```python
from build123d import *

# Parameters (mm, degrees)
F0_R     = 1.43764
F0_R_2   = 3.175
F1_DEPTH = 2.286


with BuildPart() as f1:
    # F0 (on Front) → F1 (new body)
    with BuildSketch(Plane.XZ):
        with BuildLine():
            Line((-11.43, 0), (-17.212507, -11.5316))
            ThreePointArc((-17.212507, -11.5316), (-16.638674, -19.900319), (-8.316873, -20.955))
            ThreePointArc((-8.316873, -20.955), (0, -19.152777), (8.316873, -20.955))
            ThreePointArc((8.316873, -20.955), (16.638674, -19.900319), (17.212507, -11.5316))
            Line((17.212507, -11.5316), (12.146577, -1.429014))
            ThreePointArc((12.146577, -1.429014), (12.173853, -0.810849), (12.714209, -0.509375))
            Line((12.714209, -0.509375), (33.02, -0.509375))
            ThreePointArc((33.02, -0.509375), (35.941, 2.411625), (33.02, 5.332625))
            Line((33.02, 5.332625), (8.437909, 5.332625))
            ThreePointArc((8.437909, 5.332625), (6.409691, 5.70754), (4.543451, 6.585822))
            ThreePointArc((4.543451, 6.585822), (2.379373, 7.639017), (0, 8.001))
            ThreePointArc((0, 8.001), (-0.739302, 7.953795), (-1.474639, 7.863933))
            ThreePointArc((-1.474639, 7.863933), (-7.494188, 5.250922), (-11.43, 0))
        make_face()
        with Locations((-11.8364, -15.367)):
            Circle(F0_R, mode=Mode.SUBTRACT)
        with Locations((11.8364, -15.367)):
            Circle(F0_R, mode=Mode.SUBTRACT)
        with Locations((1.27, 3.2512)):
            Circle(F0_R_2, mode=Mode.SUBTRACT)
    extrude(amount=F1_DEPTH)


solid = f1.part
```
Design review of the part built by this model. Coordinates are the model's own, in mm. A direction names the side the tool comes from. Round coordinates to 2 decimals unless told otherwise and drop trailing zeros. Write each loop counter-clockwise with the first axis right and the second up, starting at its lowest first coordinate (ties: lowest second). Pieces come first, ordered by that corner, then holes. Notation, with made-up numbers: (36.5, -32.75) -> (46.5, -32.75) arc R25 cw to (46.5, -15.75) -> close; hole circle Ø8 at (48, 88). An arc over 180 degrees is marked (long way). Answer in a Markdown table with one row per item.
Q1. To check wall thickness, follow L1, parallel to Z at x = 12, y = -0.6; L2, parallel to Z at x = 13, y = -1.5; L3, parallel to X at y = -1.9, z = -15.75. State the ranges of each line that lie inside material, in increasing order. Write a range as [from, to].
The answers:
| item | result |
|---|---|
| L1 | [-21.97, -16.8], [-13.94, 5.33] |
| L2 | [-21.87, -16.21], [-14.52, -3.13], [-0.51, 5.33] |
| L3 | [-18.43, -13.22], [-10.45, 10.45], [13.22, 18.43] |
Q2. Take a section at A-A, the plane x = 14. State the section outline as (y, z) points.
The answers:
| item | result |
|---|---|
| outline | (-2.29, -21.61) -> (0, -21.61) -> (0, -5.13) -> (-2.29, -5.13) -> close; (-2.29, -0.51) -> (0, -0.51) -> (0, 5.33) -> (-2.29, 5.33) -> close |
Q3. Clearance check with flat-ended pins moving along their axes: pin 1 Ø2.5 at (x, z) = (11.84, -15.37) entering from +Y; pin 2 Ø1.1 at (x, y) = (26, -1.5) entering from -Z. State where each tip first meets the part, or that it passes through.
The answers:
| item | result |
|---|---|
| pin 1 | through |
| pin 2 | z = -0.51 |
Q4. Take a section at C-C, the plane z = 1. State the section outline as (x, y) points, then the cut area to 3 significant figures.
The answers:
| item | result |
|---|---|
| outline | (-10.97, -2.29) -> (-0.97, -2.29) -> (-0.97, 0) -> (-10.97, 0) -> close; (3.51, -2.29) -> (35.58, -2.29) -> (35.58, 0) -> (3.51, 0) -> close |
| area | 96.2 mm² |
Q5. For faces 1 (the face through (21, -1, 5.333)), 2 (the face through (23, -1, -0.509)), 3 (the face through (-14.281, -1.127, -5.685)), list the 3-axis set-ups (+Z, -Z, +X, -X, +Y, -Y) from which the entire face can be reached by the end or side of a thin tool; tool diameter is ignored.
The answers:
| item | result |
|---|---|
| face 1 | +Z, +X, +Y, -Y |
| face 2 | +X, +Y, -Y |
| face 3 | +Z, -X, +Y, -Y |
Q6. Take a section at D-D, the plane z = -5.75. State the section outline as (x, y) points.
The answers:
| item | result |
|---|---|
| outline | (-14.31, -2.29) -> (14.31, -2.29) -> (14.31, 0) -> (-14.31, 0) -> close |
Q7. Take a section at B-B, the plane y = -0.8. Count the separate pieces of the cut face and the enclosed holes in it, then the cut area to 3 significant figures.
The answers:
| item | result |
|---|---|
| separate pieces | 1 |
| enclosed holes | 3 |
| area | 887 mm² |
Q8. Draft analysis for pull direction X (two halves, no side actions). For faces 4 (the face through (0.86, -1.13, 6.4)), 5 (the face through (2, -2.286, -7)), 6 (the face through (35.94, -1.13, 2.35)), state which applies: +X half, -X half, draft (parallel to the pull), parting line (faces both ways), or undercut.
The answers:
| item | result |
|---|---|
| face 4 | undercut |
| face 5 | draft |
| face 6 | +X half |
